Check sheet for the drawn part. Datum: minimum x, y, z corner. Units: mm. A direction names the side the tool comes from. Round coordinates to 2 decimals unless told otherwise and drop trailing zeros. Order: outer loops, then holes, each group sorted by start corner. A loop starts at its lowest first (then second) coordinate and runs counter-clockwise, first axis right, second up. Notation, with made-up numbers: M -28.5,33 L 16.5,33 A17 cw 16.5,58 Z; hole C -28,50 d2. An arc over 180 degrees is marked long. Answer as a JSON object with one key per item and string values. Group by question number.
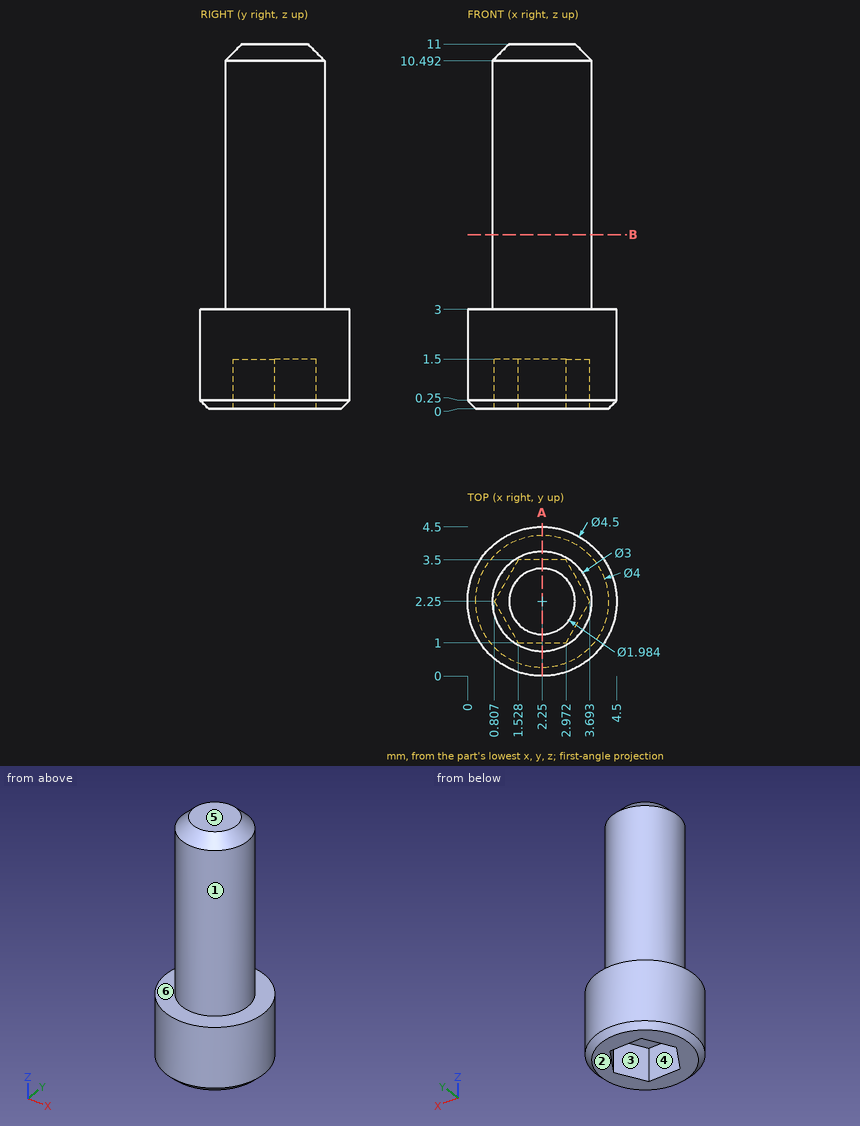
1) Sectioned sample at A-A (x = 2.25). Record the boundary of the cut face in (y, z).
2) Go/stop test with flat-tipped pins: P1, Ø2, axis at y = 1, z = 6.5, coming from the +X side; P2, Ø2, axis at y = 2, z = 9.5, coming from the -X side; P3, Ø1, axis at x = 2, z = 4.5, coming from the +Y side. Record where each tip stops, or that it passes through.
3) Thickness scan on line 1 along Z through (x, y) = (0.6, 1.85); line 2 along Z through (x, y) = (2.55, 2.3); line 3 along X through (y, z) = (2.15, 6). Record the ranges inside material, lowest first. Write a range as [from, to].
4) Set-up check for the marked faces 5 and 6: record each of +Z, -Z, +X, -X, +Y, -Y from which the full face is reachable in a straight line by a thin tool's end or side.
5) Release check for a two-part mould opening along X. For the marked faces 1, 2, 3 and 4 record: +X half, -X half, draft (parallel to the pull), parting line (faces both ways), or undercut.
6) Sectioned sample at B-B (z = 5.25). Record the boundary of the cut face in (x, y).
Final values:
{
 "1": {"outline": "M 0,0.25 L 0.25,0 L 1,0 L 1,1.5 L 3.5,1.5 L 3.5,0 L 4.25,0 L 4.5,0.25 L 4.5,3 L 3.75,3 L 3.75,10.49 L 3.24,11 L 1.26,11 L 0.75,10.49 L 0.75,3 L 0,3 Z"},
 "2": {"P1": "stops at x = 3.73", "P2": "stops at x = 0.75", "P3": "stops at y = 3.75"},
 "3": {"line 1": "z = [0, 3]", "line 2": "z = [1.5, 11]", "line 3": "x = [0.75, 3.75]"},
 "4": {"face 5": "+Z, +X, -X, +Y, -Y", "face 6": "+Z"},
 "5": {"face 1": "parting line", "face 2": "draft", "face 3": "undercut", "face 4": "undercut"},
 "6": {"outline": "C 2.25,2.25 d3"}
}
